```python
from build123d import *

# Parameters (mm, degrees)
BOSS_EXTRUDE1_DEPTH = 3.95
SKETCH2_R           = 3.575
CUT_EXTRUDE1_DEPTH  = 3.95
BOSS_EXTRUDE2_DEPTH = 1.64
SKETCH4_R           = 3.3
CUT_EXTRUDE2_DEPTH  = 31.43771091


with BuildPart() as part:
    # Sketch1 → Boss-Extrude1 (new body)
    with BuildSketch(Plane(origin=(0, 0, 0), x_dir=(1, 0, 0), z_dir=(0, 1, 0))):
        with BuildLine():
            Line((0, 7), (22.089622642, 7))
            ThreePointArc((22.089622642, 7), (29.089622642, 0), (22.089622642, -7))
            Line((22.089622642, -7), (0, -7))
            ThreePointArc((0, -7), (-7, 0), (0, 7))
        make_face()
    extrude(amount=BOSS_EXTRUDE1_DEPTH)

    # Sketch2 → Cut-Extrude1 (cut)
    with BuildSketch(Plane.XZ):
        with Locations(Location((0, 0, 0), (0, 0, 270))):
            Circle(SKETCH2_R)
    extrude(amount=-CUT_EXTRUDE1_DEPTH, mode=Mode.SUBTRACT)

    # Sketch3 → Boss-Extrude2 (add)
    with BuildSketch(Plane(origin=(0, 3.95, 0), x_dir=(1, 0, 0), z_dir=(0, 1, 0))):
        with BuildLine():
            Line((0, -7), (22.089622642, -7))
            ThreePointArc((22.089622642, -7), (29.089622642, 0), (22.089622642, 7))
            Line((22.089622642, 7), (0, 7))
            ThreePointArc((0, 7), (-7, 0), (0, -7))
        make_face()
        with BuildLine():
            Line((13.979308982, 2.569996388), (1.997926282, 3.167540934))
            ThreePointArc((1.997926282, 3.167540934), (-3.745, 0), (1.997926282, -3.167540934))
            Line((1.997926282, -3.167540934), (13.979308982, -2.569996388))
            ThreePointArc((13.979308982, -2.569996388), (16.545, 0), (13.979308982, 2.569996388))
        make_face(mode=Mode.SUBTRACT)
    extrude(amount=BOSS_EXTRUDE2_DEPTH)

    # Sketch4 → Cut-Extrude2 (cut, through all)
    with BuildSketch(Plane(origin=(0, 5.59, 0), x_dir=(1, 0, 0), z_dir=(0, 1, 0))):
        with Locations(Location((22.089622642, 0, 0), (0, 0, 270))):
            Circle(SKETCH4_R)
    extrude(amount=-CUT_EXTRUDE2_DEPTH, mode=Mode.SUBTRACT)


solid = part.part
```
Here's how the part is built. I have some questions about the finished solid (model axes, mm). A direction names the side the tool comes from. Round coordinates to 2 decimals unless told otherwise and drop trailing zeros. Loops run counter-clockwise (first coordinate to the right, second up) from the corner with the lowest first, then second, coordinate; pieces in that order, holes last.
1. Suppose I cut it at C-C, the plane y = 0.6. Please give me the cut outline in (x, z) (3 decimals).
Answers:
outline: (0, -7) - (22.09, -7) arc R7 ccw to (22.09, 7) - (0, 7) arc R7 ccw to start; hole circle Ø7.15 at (0, 0); hole circle Ø6.6 at (22.09, 0)
2. If I drill on probe 1 along X at (y, z) = (3.9, 0) (3 decimals); probe 2 along X at (y, z) = (4.9, 0) (3 decimals); probe 3 along Z at (x, y) = (22, 3.45), over which ranges is the centre line in solid material (lowest first)?
Answers:
probe 1: x = -7 to -3.575, 3.575 to 18.79, 25.39 to 29.09
probe 2: x = -7 to -3.745, 16.545 to 18.79, 25.39 to 29.09
probe 3: z = -7 to -3.3, 3.3 to 7
3. Thinking about a two-plate mould opening in X: for faces 1 (the face through (11, 3, 7)), 2 (the face through (8.072, 4.759, -2.865)), 3 (the face through (-7, 3, 0)), which applies, released by +X, released by -X, zero draft, split by the parting line, or undercut?
Answers:
face 1: zero draft
face 2: undercut
face 3: released by -X
4. For faces 4 (the face through (9, 3.95, 0)), 5 (the face through (11, 0, 0)), which set-ups out of +Z, -Z, +X, -X, +Y, -Y let a thin tool reach every point of the face, with its end or its side?
Answers:
face 4: +Y
face 5: +Z, -Z, +X, -X, -Y
5. Suppose I cut it at B-B, the plane x = 25. Please give me the cut outline in (y, z).
Answers:
outline: (0, -6.37) - (5.59, -6.37) - (5.59, -1.56) - (0, -1.56) - close; (0, 1.56) - (5.59, 1.56) - (5.59, 6.37) - (0, 6.37) - close
6. Suppose I cut it at D-D, the plane x = 9.5. Please give me the cut outline in (y, z), and give its area (3 significant figures).
Answers:
outline: (0, -7) - (5.59, -7) - (5.59, -2.79) - (3.95, -2.79) - (3.95, 2.79) - (5.59, 2.79) - (5.59, 7) - (0, 7) - close
area: 69.1 mm2
7. Will these pins go through, and if not, where does the flat tip stop? pin 1 (8 mm diameter, centred on x = 8, z = 1, fed in from +Y); pin 2 (6.5 mm diameter, centred on x = 0, z = 0, fed in from -Y); pin 3 (1 mm diameter, centred on y = 1, z = -1, fed in from +X).
Answers:
pin 1: stops at y = 5.59
pin 2: passes through
pin 3: stops at x = 29.07
8. Suppose I cut it at A-A, the plane z = 0. Please give me the cut outline in (x, y) (3 decimals), and give its area (3 significant figures).
Answers:
outline: (-7, 0) - (-3.575, 0) - (-3.575, 3.95) - (-3.745, 3.95) - (-3.745, 5.59) - (-7, 5.59) - close; (3.575, 0) - (18.79, 0) - (18.79, 5.59) - (16.545, 5.59) - (16.545, 3.95) - (3.575, 3.95) - close; (25.39, 0) - (29.09, 0) - (29.09, 5.59) - (25.39, 5.59) - close
area: 103 mm2
